Part model, mm, in its own coordinate system. A direction names the side the tool comes from. Coordinates: 2 decimals unless noted, no trailing zeros. Order: outer loops, then holes, each group sorted by start corner. A loop starts at its lowest first (then second) coordinate and runs counter-clockwise, first axis right, second up.
1) Pin check, flat tips, straight feed: pin 1 Ø2.5 at (x, y) = (40.5, 29) entering from +Z; pin 2 Ø2 at (x, y) = (-5, 25) entering from -Z; pin 3 Ø3 at (x, y) = (33.5, 35) entering from +Z. Stop position of each tip, or through.
2) Tool access for faces 1 (the flat face through (21, 30, 0.95)), 2 (the flat face through (14.5, 30, -23)), 3 (the flat face through (-7.75, 30, -12)), 4 (the flat face through (28.5, 30, 13)), 5 (the flat face through (-0.399, 27.594, 28.413)): list every direction of +Z, -Z, +X, -X, +Y, -Y with a clear straight run to the whole face (end or side of a thin tool).
3) Mould opens along Z. For faces 6 (the cylindrical face through (19.969, 43.137, 22.287)), 7 (the flat face through (0, 37.5, 22)), 8 (the flat face through (28, 30, -33.171)) say: +Z half, -Z half, draft (parallel to the pull), parting line (faces both ways), or undercut.
4) Cut at C-C (x = 26.5). Give the number of separate pieces and of enclosed holes in the cut face, and give its area (3 significant figures).
5) Wall check: L1, parallel to Y at x = 19, z = 20; L2, parallel to Z at x = 21.5, y = 21.5; L3, parallel to X at y = 52, z = -14.5. Give the ranges that are in metal, low to high.
6) Cut at B-B (z = -21). List the corners of the cut face in (x, y).
7) Cut at A-A (z = 26). List the corners of the cut face in (x, y), and give its area (3 significant figures).
```python
from build123d import *

# Parameters (mm, degrees)
SKETCH1_W           = 57
SKETCH1_H           = 28.7
BOSS_EXTRUDE1_DEPTH = 60
SKETCH2_W           = 9
SKETCH2_H           = 4
CUT_EXTRUDE1_DEPTH  = 69.064473112
BOSS_EXTRUDE2_DEPTH = 28.5
SKETCH6_W           = 15.5
SKETCH6_H           = 15.390476131
CUT_EXTRUDE2_DEPTH  = 80
BOSS_EXTRUDE5_DEPTH = 60
SKETCH10_R          = 2.1
CUT_EXTRUDE3_DEPTH  = 24.530533394
SKETCH11_W          = 40.163550966
SKETCH11_H          = 20.084690285
CUT_EXTRUDE4_DEPTH  = 82.168165413
SKETCH12_W          = 9
SKETCH12_H          = 4
BOSS_EXTRUDE6_DEPTH = 60


with BuildPart() as part:
    # Sketch1 → Boss-Extrude1 (new body)
    with BuildSketch(Plane(origin=(0, 0, 0), x_dir=(1, 0, 0), z_dir=(0, 1, 0))):
        with Locations((0, -0.5)):
            Rectangle(SKETCH1_W, SKETCH1_H)
        Polygon((23.07, -9.85), (-23.07, -9.85), (-23.5, -9.42), (-23.5, -0.95), (-19.09385128, -0.95), (-19, -0.599742255), (-16.2, 9.85), (16.2, 9.85), (19, -0.599742255), (19.09385128, -0.95), (23.5, -0.95), (23.5, -2.9), (23.5, -9.42), align=None, mode=Mode.SUBTRACT)
    extrude(amount=BOSS_EXTRUDE1_DEPTH)

    # Sketch2 → Cut-Extrude1 (cut, through all)
    with BuildSketch(Plane.XZ):
        with Locations((24, -10.0706285)):
            Rectangle(SKETCH2_W, SKETCH2_H)
        with Locations((-24, -10.0706285)):
            Rectangle(SKETCH2_W, SKETCH2_H)
    extrude(amount=-CUT_EXTRUDE1_DEPTH, mode=Mode.SUBTRACT)

    # Sketch5 → Boss-Extrude2 (add, symmetric)
    with BuildSketch(Plane(origin=(0, 0, 0), x_dir=(0, 0, -1), z_dir=(1, 0, 0))):
        with BuildLine():
            Line((-14.85, 0), (-14.85, 23.200000017))
            Line((-14.85, 23.200000017), (-15.549999973, 22.50000003))
            Line((-15.549999973, 22.50000003), (-29.149999973, 22.50000003))
            Line((-29.149999973, 22.50000003), (-29.849999973, 23.20000003))
            Line((-29.849999973, 23.20000003), (-29.849999973, 25.743360053))
            ThreePointArc((-29.849999973, 25.743360053), (-29.773879502, 26.126043492), (-29.557106746, 26.450466847))
            Line((-29.557106746, 26.450466847), (-27.237157266, 28.770416328))
            ThreePointArc((-27.237157266, 28.770416328), (-27.150448162, 28.900185674), (-27.119999973, 29.053259055))
            Line((-27.119999973, 29.053259055), (-27.119999973, 30.615319642))
            ThreePointArc((-27.119999973, 30.615319642), (-27.150448164, 30.768393021), (-27.237157268, 30.898162365))
            Line((-27.237157268, 30.898162365), (-27.431588163, 31.09259326))
            ThreePointArc((-27.431588163, 31.09259326), (-27.613507965, 31.297692563), (-27.620638933, 31.57175403))
            ThreePointArc((-27.620638933, 31.57175403), (-28.017573243, 32.42857618), (-28.828543655, 32.91234062))
            ThreePointArc((-28.828543655, 32.91234062), (-29.01918836, 33.020436377), (-29.124259054, 33.212764861))
            Line((-29.124259054, 33.212764861), (-29.156235284, 33.354092333))
            ThreePointArc((-29.156235284, 33.354092333), (-29.24659278, 33.53064407), (-29.410649592, 33.642090719))
            Line((-29.410649592, 33.642090719), (-29.585724304, 33.70524196))
            ThreePointArc((-29.585724304, 33.70524196), (-29.777329878, 33.851609246), (-29.849999973, 34.081511694))
            Line((-29.849999973, 34.081511694), (-29.849999973, 34.837490602))
            ThreePointArc((-29.849999973, 34.837490602), (-29.772088513, 35.074680338), (-29.568705112, 35.219471078))
            Line((-29.568705112, 35.219471078), (-29.427668799, 35.263299846))
            ThreePointArc((-29.427668799, 35.263299846), (-29.25116358, 35.375371369), (-29.155313737, 35.561185593))
            Line((-29.155313737, 35.561185593), (-29.125010632, 35.702102112))
            ThreePointArc((-29.125010632, 35.702102112), (-29.020526118, 35.897067182), (-28.828406063, 36.006695082))
            ThreePointArc((-28.828406063, 36.006695082), (-28.025619489, 36.481556021), (-27.62403672, 37.32339358))
            ThreePointArc((-27.62403672, 37.32339358), (-27.540484938, 37.407225271), (-27.43605838, 37.46293655))
            Line((-27.43605838, 37.46293655), (-27.39899493, 37.5))
            Line((-27.39899493, 37.5), (-17.30100503, 37.5))
            Line((-17.30100503, 37.5), (-17.26394158, 37.46293655))
            ThreePointArc((-17.26394158, 37.46293655), (-17.159515017, 37.407225278), (-17.07596324, 37.32339358))
            ThreePointArc((-17.07596324, 37.32339358), (-16.674380468, 36.481556018), (-15.871593887, 36.006695079))
            ThreePointArc((-15.871593887, 36.006695079), (-15.679473839, 35.897067189), (-15.574989331, 35.702102127))
            Line((-15.574989331, 35.702102127), (-15.544686222, 35.561185587))
            ThreePointArc((-15.544686222, 35.561185587), (-15.448836377, 35.375371364), (-15.272331158, 35.263299843))
            Line((-15.272331158, 35.263299843), (-15.131294869, 35.219471083))
            ThreePointArc((-15.131294869, 35.219471083), (-14.927911462, 35.074680333), (-14.85, 34.837490586))
            Line((-14.85, 34.837490586), (-14.85, 60))
            Line((-14.85, 60), (-34.380533394, 60))
            Line((-34.380533394, 60), (-34.380533394, 0))
            Line((-34.380533394, 0), (-14.85, 0))
        make_face()
        with BuildLine():
            ThreePointArc((-15.142893227, 26.450466847), (-14.926120471, 26.126043492), (-14.85, 25.743360053))
            Line((-14.85, 25.743360053), (-14.85, 34.081511674))
            ThreePointArc((-14.85, 34.081511674), (-14.922670087, 33.851609245), (-15.114275644, 33.70524197))
            Line((-15.114275644, 33.70524197), (-15.289350386, 33.642090718))
            ThreePointArc((-15.289350386, 33.642090718), (-15.453407192, 33.53064407), (-15.543764688, 33.354092339))
            Line((-15.543764688, 33.354092339), (-15.57574092, 33.21276486))
            ThreePointArc((-15.57574092, 33.21276486), (-15.680811613, 33.020436377), (-15.871456319, 32.91234062))
            ThreePointArc((-15.871456319, 32.91234062), (-16.68242673, 32.42857618), (-17.07936104, 31.57175403))
            ThreePointArc((-17.07936104, 31.57175403), (-17.086492012, 31.297692565), (-17.26841181, 31.09259326))
            Line((-17.26841181, 31.09259326), (-17.462842708, 30.898162362))
            ThreePointArc((-17.462842708, 30.898162362), (-17.549551812, 30.768393016), (-17.58, 30.615319635))
            Line((-17.58, 30.615319635), (-17.58, 29.053259048))
            ThreePointArc((-17.58, 29.053259048), (-17.54955181, 28.900185669), (-17.462842705, 28.770416325))
            Line((-17.462842705, 28.770416325), (-15.142893227, 26.450466847))
        make_face()
    extrude(amount=BOSS_EXTRUDE2_DEPTH, both=True)

    # Sketch6 → Cut-Extrude2 (cut)
    with BuildSketch(Plane(origin=(0, 60, 0), x_dir=(1, 0, 0), z_dir=(0, 1, 0))):
        with Locations((0, 12.050145064)):
            Rectangle(SKETCH6_W, SKETCH6_H)
    extrude(amount=-CUT_EXTRUDE2_DEPTH, mode=Mode.SUBTRACT)

    # Sketch9 → Boss-Extrude5 (add)
    with BuildSketch(Plane(origin=(0, 60, 0), x_dir=(1, 0, 0), z_dir=(0, 1, 0))):
        Polygon((-19.5, 13.85), (-19.5, 29.1706285), (-37.5, 29.1706285), (-37.5, 13.85), (-42.5, 13.85), (-42.5, 33.1706285), (-14.5, 33.1706285), (-14.5, 13.85), align=None)
        Polygon((37.5, 13.85), (37.5, 29.1706285), (19.5, 29.1706285), (19.5, 13.85), (14.5, 13.85), (14.5, 33.1706285), (42.5, 33.1706285), (42.5, 13.85), align=None)
    extrude(amount=-BOSS_EXTRUDE5_DEPTH)

    # Sketch10 → Cut-Extrude3 (cut)
    with BuildSketch(Plane.XY.offset(34.380533394)):
        with Locations((-19, 45)):
            Circle(SKETCH10_R)
        with Locations((19, 45)):
            Circle(SKETCH10_R)
        with Locations((-19, 15)):
            Circle(SKETCH10_R)
        with Locations((19, 15)):
            Circle(SKETCH10_R)
    extrude(amount=-CUT_EXTRUDE3_DEPTH, mode=Mode.SUBTRACT)

    # Sketch11 → Cut-Extrude4 (cut, through all)
    with BuildSketch(Plane.XZ):
        with Locations((-27.831775483, -23.892345143)):
            Rectangle(SKETCH11_W, SKETCH11_H)
    extrude(amount=-CUT_EXTRUDE4_DEPTH, mode=Mode.SUBTRACT)

    # Sketch12 → Boss-Extrude6 (add, through all)
    with BuildSketch(Plane(origin=(0, 0, 0), x_dir=(-1, 0, 0), z_dir=(0, -1, 0))):
        with Locations((24, 10.0706285)):
            Rectangle(SKETCH12_W, SKETCH12_H)
    extrude(amount=-BOSS_EXTRUDE6_DEPTH)


solid = part.part
```
Geometry check:
1. pin 1: stops at z = -13.85
1. pin 2: stops at z = 9.85
1. pin 3: stops at z = -29.17
2. face 1: +Y, -Y
2. face 2: -Z, -X, +Y, -Y
2. face 3: -Z, +Y, -Y
2. face 4: +Z, +X, +Y, -Y
2. face 5: +X, -X
3. face 6: draft
3. face 7: undercut
3. face 8: -Z half
4. separate pieces: 3
4. enclosed holes: 1
4. area: 2,700 mm2
5. L1: y = 0 to 12.9, 17.1 to 22.5, 37.5 to 42.9, 47.1 to 60
5. L2: z = -33.17 to -29.17, -13.85 to -12.07, -8.07 to 0.95, 9.85 to 34.38
5. L3: x = 14.5 to 19.5, 37.5 to 42.5
6. outline: (14.5, 0) - (19.5, 0) - (19.5, 60) - (14.5, 60) - close; (37.5, 0) - (42.5, 0) - (42.5, 60) - (37.5, 60) - close
7. outline: (-28.5, 0) - (28.5, 0) - (28.5, 22.5) - (-28.5, 22.5) - close; (-28.5, 37.5) - (28.5, 37.5) - (28.5, 60) - (-28.5, 60) - close; hole circle Ø4.2 at (-19, 15); hole circle Ø4.2 at (-19, 45); hole circle Ø4.2 at (19, 15); hole circle Ø4.2 at (19, 45)
7. area: 2,510 mm2
